Check sheet for the modelled part. Datum: model origin and axes. Units: mm. A direction names the side the tool comes from. Round coordinates to 2 decimals unless told otherwise and drop trailing zeros. Order: outer loops, then holes, each group sorted by start corner. A loop starts at its lowest first (then second) coordinate and runs counter-clockwise, first axis right, second up. Notation, with made-up numbers: M 10.25,75.25 L 51.25,75.25 A10 ccw 51.25,88.25 Z; hole C 24.25,-9.5 d8. An arc over 180 degrees is marked long. One line per item, written item: value. Start each with the question number.
(1) Cross-section at C-C, the plane y = 4. Enter the section's corners in (x, z), and give its area (3 significant figures).
(2) Cross-section at D-D, the plane z = -19.05. Enter the section's corners in (x, y).
(3) Depth check by flat-ended pin: pin 1 Ø7.5 at (y, z) = (19.05, -44.45) entering from +X; pin 2 Ø6 at (x, y) = (-16.5, 26) entering from +Z; pin 3 Ø4 at (x, z) = (-27, -30.5) entering from -Y. Enter the tip coordinate at first touch or a pass-through.
(4) Cross-section at A-A, the plane x = -25.4. Count the separate pieces of the cut face and the enclosed holes in it, and give its area (3 significant figures).
(5) Cross-section at B-B, the plane y = 12. Enter the section's corners in (x, z), and give its area (3 significant figures).
(6) Release check for a two-part mould opening along X. For faces 4 (the face through (-37.846, 20, -32)), 5 (the face through (-25.35, 26.05, -6.26)), 6 (the face through (-0.764, 0.724, -32.194)), 7 (the face through (-50.8, 18, -32)) record: released by +X, released by -X, zero draft, split by the parting line, or undercut.
(7) Thickness scan on L1, parallel to Z at x = -37.5, y = 19; L2, parallel to X at y = 9, z = -50.5; L3, parallel to X at y = 24, z = -31.5. Record the ranges inside material, lowest first.
(8) Access from +Z, -Z, +X, -X, +Y, -Y to the whole of each face (thin tool, end or side, straight path). Record for faces 1 (the face through (-25, 3, -38.608)), 2 (the face through (-28.78, 19.61, -33.51)), 3 (the face through (-10, 7.62, -32)).
from build123d import *

# Parameters (mm, degrees)
SKETCH1_W           = 63.5
SKETCH1_H           = 6.35
BOSS_EXTRUDE1_DEPTH = 50.8
BOSS_EXTRUDE2_DEPTH = 50.8
SKETCH10_W          = 6.858
SKETCH10_H          = 25.629031657
CUT_EXTRUDE1_DEPTH  = 88.854357354
LPATTERN3_COUNT     = 2
LPATTERN3_PITCH     = 31.496
SKETCH11_R          = 4.7625
CUT_EXTRUDE2_DEPTH  = 88.854357354
FILLET1_R           = 2.54
SKETCH24_R          = 3.81
CUT_EXTRUDE10_DEPTH = 88.854357354
CUT_EXTRUDE11_DEPTH = 6.35


with BuildPart() as part:
    # Sketch1 → Boss-Extrude1 (new body)
    with BuildSketch(Plane(origin=(0, 0, 0), x_dir=(0, 0, -1), z_dir=(1, 0, 0))):
        with Locations((31.75, 3.175)):
            Rectangle(SKETCH1_W, SKETCH1_H)
    extrude(amount=-BOSS_EXTRUDE1_DEPTH)

    # Sketch2 → Boss-Extrude2 (add)
    with BuildSketch(Plane(origin=(0, 0, 0), x_dir=(0, 0, -1), z_dir=(1, 0, 0))):
        Polygon((0, 6.35), (0, 19.05), (12.7, 33.249031657), (50.8, 33.249031657), (63.5, 19.05), (63.5, 6.35), align=None)
    extrude(amount=-BOSS_EXTRUDE2_DEPTH)

    # Sketch10 → Cut-Extrude1 (cut, through all)
    with BuildSketch(Plane(origin=(0, 0, -63.5), x_dir=(-1, 0, 0), z_dir=(0, 0, -1))):
        with Locations((9.779, 20.434515829)):
            Rectangle(SKETCH10_W, SKETCH10_H)
    cut_extrude1 = extrude(amount=-CUT_EXTRUDE1_DEPTH, mode=Mode.SUBTRACT)

    # LPattern3: Cut-Extrude1 ×2
    with Locations(*[(-i * LPATTERN3_PITCH, 0, 0) for i in range(1, LPATTERN3_COUNT)]):
        add(cut_extrude1, mode=Mode.SUBTRACT)

    # Sketch11 → Cut-Extrude2 (cut, through all)
    with BuildSketch(Plane(origin=(0, 0, 0), x_dir=(0, 0, -1), z_dir=(1, 0, 0))):
        with Locations((19.05, 19.05)):
            Circle(SKETCH11_R)
        with Locations((44.45, 19.05)):
            Circle(SKETCH11_R)
    extrude(amount=-CUT_EXTRUDE2_DEPTH, mode=Mode.SUBTRACT)

    # Fillet1
    fillet1_edges = [part.edges().sort_by_distance(p)[0] for p in [
        (0, 0, -31.75),
        (-50.8, 0, -31.75),
        (-25.4, 0, -63.5),
        (-25.4, 0, 0),
    ]]
    fillet(fillet1_edges, radius=FILLET1_R)

    # Sketch24 → Cut-Extrude10 (cut, through all)
    with BuildSketch(Plane.XZ):
        with Locations(Location((-25.4, -31.75, 0), (0, 0, 270))):
            Circle(SKETCH24_R)
    extrude(amount=-CUT_EXTRUDE10_DEPTH, mode=Mode.SUBTRACT)

    # Sketch25 → Cut-Extrude11 (cut)
    with BuildSketch(Plane.XZ):
        Polygon((-29.359468146, -24.892), (-33.318936292, -31.75), (-29.359468146, -38.608), (-21.440531854, -38.608), (-17.481063708, -31.75), (-21.440531854, -24.892), align=None)
    extrude(amount=-CUT_EXTRUDE11_DEPTH, mode=Mode.SUBTRACT)


solid = part.part
Values found:
1. outline: M -50.8,-63.5 L 0,-63.5 L 0,0 L -50.8,0 Z; hole M -33.32,-31.75 L -29.36,-38.61 L -21.44,-38.61 L -17.48,-31.75 L -21.44,-24.89 L -29.36,-24.89 Z
1. area: 3,060 mm^2
2. outline: M -50.8,2.54 A2.54 ccw -48.26,0 L -2.54,0 A2.54 ccw 0,2.54 L 0,14.29 L -6.35,14.29 L -6.35,7.62 L -13.21,7.62 L -13.21,14.29 L -37.85,14.29 L -37.85,7.62 L -44.7,7.62 L -44.7,14.29 L -50.8,14.29 Z; M -50.8,23.81 L -44.7,23.81 L -44.7,33.25 L -50.8,33.25 Z; M -37.85,23.81 L -13.21,23.81 L -13.21,33.25 L -37.85,33.25 Z; M -6.35,23.81 L 0,23.81 L 0,33.25 L -6.35,33.25 Z
3. pin 1: through
3. pin 2: z = -3.53
3. pin 3: y = 6.35
4. separate pieces: 2
4. enclosed holes: 2
4. area: 1,490 mm^2
5. outline: M -50.8,-63.5 L -44.7,-63.5 L -44.7,0 L -50.8,0 Z; M -37.85,-63.5 L -13.21,-63.5 L -13.21,0 L -37.85,0 Z; M -6.35,-63.5 L 0,-63.5 L 0,0 L -6.35,0 Z; hole C -25.4,-31.75 d7.62
5. area: 2,310 mm^2
6. face 4: undercut
6. face 5: zero draft
6. face 6: released by +X
6. face 7: released by -X
7. L1: -63.5 to -49.21, -39.69 to -23.81, -14.29 to 0
7. L2: -50.8 to -44.7, -37.85 to -13.21, -6.35 to 0
7. L3: -50.8 to -44.7, -37.85 to -29.2, -21.6 to -13.21, -6.35 to 0
8. face 1: -Y
8. face 2: +Y, -Y
8. face 3: +Z, -Z, +Y
